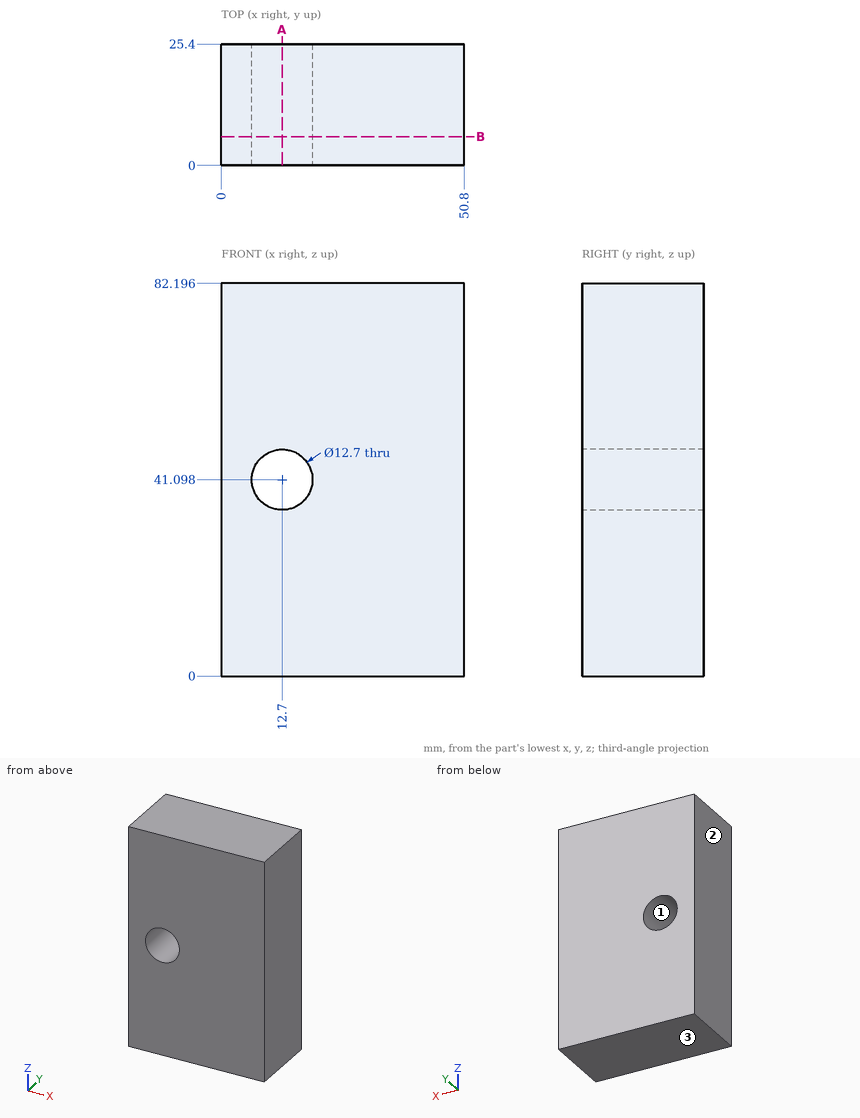
Design review of the part shown in the three views and the two pictorial views. Dimensions are in mm from the part's minimum x, y and z. Round coordinates to 2 decimals unless told otherwise and drop trailing zeros. Write each loop counter-clockwise with the first axis right and the second up, starting at its lowest first coordinate (ties: lowest second). Pieces come first, ordered by that corner, then holes.
Item 1: Consider section B-B on y = 6. Give the boundary of the cut face in (x, z), and give its area (3 significant figures).
Item 2: Draft analysis for pull direction X (two halves, no side actions). For the marked faces 1, 2 and 3, state which applies: released by +X, released by -X, zero draft, split by the parting line, or undercut.
Item 3: Consider section A-A on x = 12.7. Give the boundary of the cut face in (y, z).
Item 4: For pin 1 Ø1 at (x, z) = (25, 58) entering from -Y, flat-tipped, find the tip position at first contact; note if it passes through.
Item 5: Wall thickness on L1, parallel to Z at x = 12.7, y = 19.5; L2, parallel to X at y = 18, z = 41; L3, parallel to Z at x = 17, y = 10.75 (1 decimal): over which ranges is each line inside the solid? List them lowest first.
Check values:
1. outline: (0, 0) - (50.8, 0) - (50.8, 82.2) - (0, 82.2) - close; hole circle Ø12.7 at (12.7, 41.1)
1. area: 4,050 mm2
2. face 1: undercut
2. face 2: released by -X
2. face 3: zero draft
3. outline: (0, 0) - (25.4, 0) - (25.4, 34.75) - (0, 34.75) - close; (0, 47.45) - (25.4, 47.45) - (25.4, 82.2) - (0, 82.2) - close
4. pin 1: stops at y = 0
5. L1: z = 0 to 34.75, 47.45 to 82.2
5. L2: x = 0 to 6.35, 19.05 to 50.8
5. L3: z = 0 to 36.4, 45.8 to 82.2
